Read the model definition and answer for the solid it produces. Units are mm, in the model's axes. Face numbers are marked on the shaded views. A direction names the side the tool comes from. Give positions to 0.01 mm unless a question says otherwise; leave off trailing zeros. Order: outer loops, then holes, each group sorted by start corner. A loop starts at its lowest first (then second) coordinate and runs counter-clockwise, first axis right, second up. Notation, with made-up numbers: M 31,-11 L 60,-11 A15 ccw 60,10 Z; hole C 59.5,51 d4. An arc over 180 degrees is marked long. Write item = value, one per line. Start each with the question number.
Autodesk Inventor part; units mm, degrees
ref_plane "YZ Plane" through (0, 0, 0) normal (1, 0, 0) x (0, 1, 0)
ref_plane "XZ Plane" through (0, 0, 0) normal (0, 1, 0) x (-1, 0, 0)
ref_plane "XY Plane" through (0, 0, 0) normal (0, 0, 1) x (1, 0, 0)
sketch "草圖1" plane through (0, 0, 0) normal (0, 1, 0) x (-1, 0, 0)
  line L0 (18, 21) -> (-18, 21)
  line L1 (-21, 18) -> (-21, -18)
  line L2 (-18, -21) -> (18, -21)
  line L3 (21, -18) -> (21, 18)
  line L4 (21, 21) -> (-21, -21) construction
  line L5 (-21, 21) -> (21, -21) construction
  line L6 (21, -18) -> (18, -21)
  line L7 (-18, -21) -> (-21, -18)
  line L8 (-21, 18) -> (-18, 21)
  line L9 (18, 21) -> (21, 18)
  point P0 (0, 0)
  dimension "d0" = 42
  dimension "d1" = 42
  dimension "d2" = 3
  dimension "d3" = 3
  dimension "d4" = 3
  dimension "d5" = 3
  dimension "d6" = 3
  dimension "d7" = 3
  dimension "d8" = 3
  dimension "d9" = 3
extrude "擠出1" add sketch "草圖1" along normal blind 65
sketch "草圖2" plane through (0, 65, 0) normal (0, 1, 0) x (1, 0, 0)
  circle A0 centre (0, 0) radius 18
  dimension "d12" = 36
extrude "擠出2" add sketch "草圖2" along normal blind 36
sketch "草圖3" plane through (0, 101, 0) normal (0, 1, 0) x (1, 0, 0)
  circle A0 centre (0, 0) radius 14 construction
  circle A1 centre (0, 0) radius 11
  line L0 (0, 0) -> (-19.5, -19.5) construction
  line L1 (-21, -18) -> (-18, -21)
  circle A2 centre (-9.8995, -9.8995) radius 1.5
  circle A3 centre (9.8995, -9.8995) radius 1.5
  circle A4 centre (9.8995, 9.8995) radius 1.5
  circle A5 centre (-9.8995, 9.8995) radius 1.5
  dimension "d15" = 28
  dimension "d16" = 22
  dimension "d18" = 3
  dimension "d21" = 360
extrude "擠出3" cut sketch "草圖3" against normal blind 6 contours A2 | A3 | A4 | A5
extrude "擠出4" add sketch "草圖3" along normal blind 2 contours A1
sketch "草圖4" plane through (0, 103, 0) normal (0, 1, 0) x (1, 0, 0)
  circle A0 centre (0, 0) radius 4
  dimension "d27" = 8
extrude "擠出5" add sketch "草圖4" along normal blind 17
sketch "草圖5" plane through (0, 120, 0) normal (0, 1, 0) x (1, 0, 0)
  circle A0 centre (0, 0) radius 4
  line L0 (-3, -2.6458) -> (-3, 2.6458)
  dimension "d30" = 7
extrude "擠出6" cut sketch "草圖5" against normal blind 15 contours L0 A0 picked at (-3.1815, -0.6179)
sketch "草圖7" plane through (0, 0, 0) normal (0, -1, 0) x (1, 0, 0)
  point P0 (0, 0)
  point P1 (0, 0)
equation "\"d3\" = d2"
equation "\"d4\" = d2"
equation "\"d5\" = d4"
equation "\"d6\" = d2"
equation "\"d7\" = d6"
equation "\"d8\" = d2"
equation "\"d9\" = d8"
properties part number "stepper 42-27"
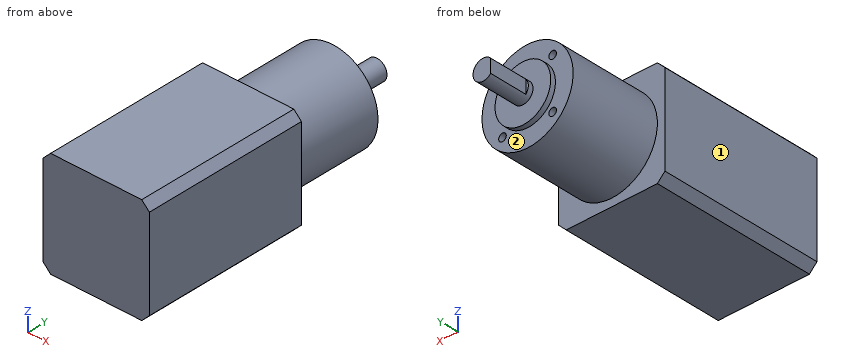
1) Find the intervals of material crossed by probe 1 along Y at (x, z) = (-16.5, 11.5); probe 2 along Y at (x, z) = (-14.5, 3.5); probe 3 along Z at (x, y) = (-16, 88), in increasing order. Write a range as [from, to].
2) Each of these flat-tipped pins is pushed along its axis until it touches: P1, Ø0.9, axis at x = 10.5, z = 9.5, coming from the +Y side; P2, Ø0.5, axis at x = -3.5, z = 0, coming from the +Y side; P3, Ø3.5, axis at x = 9.9, z = -9.9, coming from the +Y side. Where does it stop, or does it pass through?
3) Find section A-A on x = 0. Determine the outline of the cut face in (y, z).
4) Find section C-C on y = 82.5. Determine the outline of the cut face in (x, z), plus the area to 3 significant figures.
5) For the marked faces 1 and 2, determine the directions among +Z, -Z, +X, -X, +Y, -Y from which every point of the face is accessible in a straight line to the end or side of a thin tool.
6) Find section B-B on z = 0. Determine the outline of the cut face in (x, y), plus the area to 3 significant figures.
Numbers:
q1.probe_1 = [0, 65]
q1.probe_2 = [0, 101]
q1.probe_3 = [-8.25, 8.25]
q2.P1 = 95
q2.P2 = 105
q2.P3 = 101
q3.outline = M 0,-21 L 65,-21 L 65,-18 L 101,-18 L 101,-11 L 103,-11 L 103,-4 L 120,-4 L 120,4 L 103,4 L 103,11 L 101,11 L 101,18 L 65,18 L 65,21 L 0,21 Z
q4.outline = C 0,0 d36
q4.area = 1,020 mm2
q5.face_1 = +Z, -Z, -X, +Y, -Y
q5.face_2 = +Y
q6.outline = M -21,0 L 21,0 L 21,65 L 18,65 L 18,101 L 11,101 L 11,103 L 4,103 L 4,120 L -3,120 L -3,105 L -4,105 L -4,103 L -11,103 L -11,101 L -18,101 L -18,65 L -21,65 Z
q6.area = 4,190 mm2
